Part model, mm, in its own coordinate system. A direction names the side the tool comes from. Round coordinates to 2 decimals unless told otherwise and drop trailing zeros. Write each loop counter-clockwise with the first axis right and the second up, starting at its lowest first coordinate (ties: lowest second). Pieces come first, ordered by that corner, then holes. Notation, with made-up numbers: M -28,71 L 21,71 A19 ccw 21,77 Z; hole C -36.5,-7 d4. An arc over 180 degrees is marked long. Use a Markdown table: item, result. Add a question column.
1) Slice it at D-D on z = 28. Write the cut outline in (x, y), plus the area to 3 significant figures.
2) Two-plate mould, pull along X, no slides. Class faces 1 (the face through (31.2, -11.7, 2.3)), 2 (the face through (24, -13, 4.572)), 3 (the face through (-18.922, -13, 11)): released by +X, released by -X, zero draft, split by the parting line, or undercut.
3) Slice it at A-A on y = -18.5. Write the cut outline in (x, z), plus the area to 3 significant figures.
4) Wall check: probe 1 along X at (y, z) = (-2.25, 7.5); probe 2 along X at (y, z) = (-8, 4); probe 3 along Z at (x, y) = (-23, -6). Give the ranges that are in metal, low to high.
5) Slice it at C-C on y = -12.7. Write the cut outline in (x, z), plus the area to 3 significant figures.
6) Drop flat-ended pins along their axis: P1, Ø12, axis at y = -7, z = 22, coming from the -X side; P2, Ø11, axis at x = 27.922, y = -12.7, coming from the +Z side; P3, Ø5, axis at y = -15, z = 12.5, coming from the +X side. Give the stop position or say it passes through.
7) Which spindle directions (+Z, -Z, +X, -X, +Y, -Y) get a long thin tool onto all of the face, cutting with end or side? Do faces 4 (the face through (-24, -13, 4.572)), 5 (the face through (-14.35, -13, 7)), 6 (the face through (18.922, -13, 11)). Say none if no direction does.
8) Slice it at B-B on z = 19. Write the cut outline in (x, y), plus the area to 3 significant figures.
```python
from build123d import *

# Parameters (mm, degrees)
F2_DEPTH = 25.4
F3_R     = 1
F4_R     = 5
F5_R     = 3.429
F6_DEPTH = 4.573


with BuildPart() as f2:
    # F1 (on Front) → F2 (new body)
    with BuildSketch(Plane.XZ):
        with BuildLine():
            ThreePointArc((0, 28.7), (10.14698231, 24.49698231), (14.35, 14.35))
            Line((14.35, 14.35), (14.35, 0))
            Line((14.35, 0), (35.922, 0))
            Line((35.922, 0), (35.922, 4.572))
            Line((35.922, 4.572), (18.922, 4.572))
            Line((18.922, 4.572), (18.922, 15.572))
            ThreePointArc((18.922, 15.572), (12.9685102335, 28.1830441452), (0, 33.3114178795))
            ThreePointArc((0, 33.3114178795), (-12.9685102335, 28.1830441452), (-18.922, 15.572))
            Line((-18.922, 15.572), (-18.922, 4.572))
            Line((-18.922, 4.572), (-35.922, 4.572))
            Line((-35.922, 4.572), (-35.922, 0))
            Line((-35.922, 0), (-14.35, 0))
            Line((-14.35, 0), (-14.35, 14.35))
            ThreePointArc((-14.35, 14.35), (-10.14698231, 24.49698231), (0, 28.7))
        make_face()
    extrude(amount=F2_DEPTH)

    # F3
    f3_edges = [f2.edges().sort_by_distance(p)[0] for p in [
        (-18.922, -12.7, 4.572),
        (18.922, -12.7, 4.572),
    ]]
    fillet(f3_edges, radius=F3_R)

    # F4
    f4_edges = [f2.edges().sort_by_distance(p)[0] for p in [
        (-35.922, -25.4, 2.286),
        (35.922, -25.4, 2.286),
        (35.922, 0, 2.286),
        (-35.922, 0, 2.286),
    ]]
    fillet(f4_edges, radius=F4_R)

    # F5 (on face) → F6 (cut, through all)
    with BuildSketch(Plane.XY.offset(4.572)):
        with Locations((-27.922, -12.7)):
            Circle(F5_R)
        with Locations((27.922, -12.7)):
            Circle(F5_R)
    extrude(amount=-F6_DEPTH, mode=Mode.SUBTRACT)


solid = f2.part
```
Entries:
| question | item | result |
|---|---|---|
| 1 | outline | M -13.16,-25.4 L -4.43,-25.4 L -4.43,0 L -13.16,0 Z; M 4.43,-25.4 L 13.16,-25.4 L 13.16,0 L 4.43,0 Z |
| 1 | area | 444 mm^2 |
| 2 | face 1 | undercut |
| 2 | face 2 | zero draft |
| 2 | face 3 | released by -X |
| 3 | outline | M -35.92,0 L -14.35,0 L -14.35,14.35 A14.35 cw 14.35,14.35 L 14.35,0 L 35.92,0 L 35.92,4.57 L 19.92,4.57 A1 cw 18.92,5.57 L 18.92,15.57 A18.96 ccw -18.92,15.57 L -18.92,5.57 A1 cw -19.92,4.57 L -35.92,4.57 Z |
| 3 | area | 528 mm^2 |
| 4 | probe 1 | x = -18.92 to -14.35, 14.35 to 18.92 |
| 4 | probe 2 | x = -35.92 to -14.35, 14.35 to 35.92 |
| 4 | probe 3 | z = 0 to 4.57 |
| 5 | outline | M -35.92,0 L -31.35,0 L -31.35,4.57 L -35.92,4.57 Z; M -24.49,0 L -14.35,0 L -14.35,14.35 A14.35 cw 14.35,14.35 L 14.35,0 L 24.49,0 L 24.49,4.57 L 19.92,4.57 A1 cw 18.92,5.57 L 18.92,15.57 A18.96 ccw -18.92,15.57 L -18.92,5.57 A1 cw -19.92,4.57 L -24.49,4.57 Z; M 31.35,0 L 35.92,0 L 35.92,4.57 L 31.35,4.57 Z |
| 5 | area | 466 mm^2 |
| 6 | P1 | stops at x = -18.89 |
| 6 | P2 | stops at z = 4.57 |
| 6 | P3 | stops at x = 18.92 |
| 7 | face 4 | +Z, -X, +Y, -Y |
| 7 | face 5 | -Z, +Y, -Y |
| 7 | face 6 | +Z, +X, +Y, -Y |
| 8 | outline | M -18.38,-25.4 L -13.58,-25.4 L -13.58,0 L -18.38,0 Z; M 13.58,-25.4 L 18.38,-25.4 L 18.38,0 L 13.58,0 Z |
| 8 | area | 244 mm^2 |
